Source: CAD feature listing. Evaluate the final solid. Frame: model axes, mm. Face numbers are marked on the shaded views. A direction names the side the tool comes from. Give positions to 0.01 mm unless a question says otherwise; leave off trailing zeros. Write each loop counter-clockwise with the first axis right and the second up, starting at its lowest first coordinate (ties: lowest second). Pieces come first, ordered by that corner, then holes. Notation, with made-up numbers: M 10,7 L 53,7 A12 cw 53,21 Z; hole C 58,-38 d4. An arc over 180 degrees is marked long. Answer as a JSON object with one key per item and string values. Group by question number.
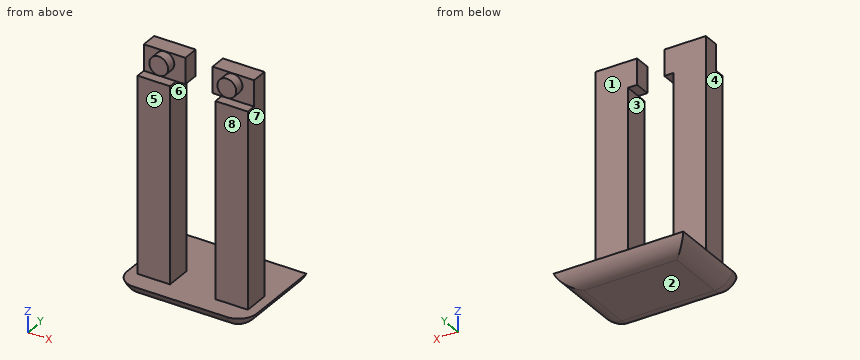
```python
from build123d import *

# Parameters (mm, degrees)
SKETCH1_W             = 50.8
SKETCH1_H             = 38.1
BOSS_EXTRUDE1_DEPTH   = 5.08
SKETCH2_W             = 16.51
SKETCH2_H             = 10.16
BOSS_EXTRUDE2_DEPTH   = 76.2
SKETCH3_W             = 3.81
SKETCH3_H             = 10.16
CUT_EXTRUDE1_DEPTH    = 76.2
SKETCH4_W             = 16.51
SKETCH4_H             = 10.16
BOSS_EXTRUDE3_DEPTH   = 12.7
SKETCH6_W             = 16.51
SKETCH6_H             = 12.7
CUT_EXTRUDE2_DEPTH    = 3.81
SKETCH5_R             = 3.683
BOSS_EXTRUDE4_DEPTH   = 3.81
FILLET1_R             = 7.62
FILLET4_R             = 7.62
FILLET7_R             = 7.62
SKETCH7_W             = 16.51
SKETCH7_H             = 6.35
LEDGE_REDUCTION_DEPTH = 2.54
SKETCH8_W             = 10.16
SKETCH8_H             = 6.35
CUT_EXTRUDE4_DEPTH    = 0.254
SKETCH9_W             = 10.16
SKETCH9_H             = 6.35
CUT_EXTRUDE5_DEPTH    = 0.254


with BuildPart() as part:
    # Sketch1 → Boss-Extrude1 (new body)
    with BuildSketch(Plane.XY):
        Rectangle(SKETCH1_W, SKETCH1_H)
    extrude(amount=BOSS_EXTRUDE1_DEPTH)

    # Sketch2 → Boss-Extrude2 (add)
    with BuildSketch(Plane.XY.offset(5.08)):
        with Locations((-13.335, -5.842)):
            Rectangle(SKETCH2_W, SKETCH2_H)
        with Locations((13.335, -5.842)):
            Rectangle(SKETCH2_W, SKETCH2_H)
    extrude(amount=BOSS_EXTRUDE2_DEPTH)

    # Sketch3 → Cut-Extrude1 (cut)
    with BuildSketch(Plane.XY.offset(81.28)):
        with Locations((-6.985, -5.842)):
            Rectangle(SKETCH3_W, SKETCH3_H)
        with Locations((6.985, -5.842)):
            Rectangle(SKETCH3_W, SKETCH3_H)
    extrude(amount=-CUT_EXTRUDE1_DEPTH, mode=Mode.SUBTRACT)

    # Sketch4 → Boss-Extrude3 (add)
    with BuildSketch(Plane.XY.offset(81.28)):
        with Locations((-13.335, -5.842)):
            Rectangle(SKETCH4_W, SKETCH4_H)
        with Locations((13.335, -5.842)):
            Rectangle(SKETCH4_W, SKETCH4_H)
    extrude(amount=BOSS_EXTRUDE3_DEPTH)

    # Sketch6 → Cut-Extrude2 (cut)
    with BuildSketch(Plane.XZ.offset(10.922)):
        with Locations((-13.335, 87.63)):
            Rectangle(SKETCH6_W, SKETCH6_H)
        with Locations((13.335, 87.63)):
            Rectangle(SKETCH6_W, SKETCH6_H)
    extrude(amount=-CUT_EXTRUDE2_DEPTH, mode=Mode.SUBTRACT)

    # Sketch5 → Boss-Extrude4 (add)
    with BuildSketch(Plane.XZ.offset(10.922)):
        with Locations(Location((-13.335, 87.63, 0), (0, 0, 270))):
            Circle(SKETCH5_R)
        with Locations(Location((13.335, 87.63, 0), (0, 0, 270))):
            Circle(SKETCH5_R)
    extrude(amount=-BOSS_EXTRUDE4_DEPTH)

    # Fillet1
    # the kernel refuses this fillet: 7.62 mm, written as the material it takes off along each edge
    with BuildSketch(Plane(origin=(-43.360512242, 19.05, 0), x_dir=(0, -1, 0), z_dir=(1, 0, 0))) as fillet1_piece_1:
        with BuildLine():
            CenterArc((7.184204897, -7.62), FILLET1_R, 90, 70.528779366)
            Line((0, -5.08), (-0.143684098, -5.0292))
            ThreePointArc((-0.143684098, -5.0292), (-0.1524, -2.54), (-0.1524, 0))
            Line((-0.1524, 0), (0, 0.1524))
            Line((0, 0.1524), (7.184204897, 0.1524))
            Line((7.184204897, 0.1524), (7.184204897, 0))
        make_face()
    extrude(amount=86.721024484, mode=Mode.SUBTRACT)

    # Fillet4
    # the kernel refuses this fillet: 7.62 mm, written as the material it takes off along each edge
    with BuildSketch(Plane(origin=(-25.4, -37.010512242, 0), x_dir=(0, 0, 1), z_dir=(0, 1, 0)), Plane(origin=(25.4, 29.826307345, 0), x_dir=(0, 0, 1), z_dir=(0, -1, 0))) as fillet4_piece_1:
        with BuildLine():
            CenterArc((7.62, 7.184204897), FILLET4_R, 180, 70.528779366)
            Line((0, 7.184204897), (-0.1524, 7.184204897))
            Line((-0.1524, 7.184204897), (-0.1524, 0))
            Line((-0.1524, 0), (0, -0.1524))
            ThreePointArc((0, -0.1524), (2.54, -0.1524), (5.0292, -0.143684098))
            Line((5.0292, -0.143684098), (5.08, 0))
        make_face()
    extrude(amount=66.836819587, mode=Mode.SUBTRACT)

    # Fillet7
    # the kernel refuses this fillet: 7.62 mm, written as the material it takes off along each edge
    with BuildSketch(Plane(origin=(-18.215795103, -19.05, 7.62), x_dir=(0.5563472554155052, 0, 0.8309498970405103), z_dir=(0.8309498970405103, 0, -0.5563472554155052))) as fillet7_piece_1:
        with BuildLine():
            CenterArc((7.62 - FILLET7_R, -FILLET7_R), FILLET7_R, 0, 90)
            Line((7.62, -FILLET7_R), (7.62, 0))
            Line((7.62, 0), (7.62 - FILLET7_R, 0))
        make_face()
    revolve(axis=Axis((-18.215795103, -19.05, 7.62), (0, -1, 0)), revolution_arc=213.803560609, mode=Mode.SUBTRACT)
    with BuildSketch(Plane(origin=(18.215795103, -19.05, 7.62), x_dir=(-0.5563472554155037, 0, 0.8309498970405114), z_dir=(-0.8309498970405114, 0, -0.5563472554155037))) as fillet7_piece_2:
        with BuildLine():
            CenterArc((7.62 - FILLET7_R, FILLET7_R), FILLET7_R, 270, 90)
            Line((7.62, FILLET7_R), (7.62, 0))
            Line((7.62, 0), (7.62 - FILLET7_R, 0))
        make_face()
    revolve(axis=Axis((18.215795103, -19.05, 7.62), (0, 1, 0)), revolution_arc=213.803560609, mode=Mode.SUBTRACT)
    with BuildSketch(Plane(origin=(18.215795103, -19.05, 0), x_dir=(0, 0, 1), z_dir=(-1, 0, 0))) as fillet7_piece_3:
        with BuildLine():
            CenterArc((FILLET7_R, FILLET7_R), FILLET7_R, 180, 90)
            Line((0, FILLET7_R), (0, 0))
            Line((0, 0), (FILLET7_R, 0))
        make_face()
    extrude(amount=36.431590206, mode=Mode.SUBTRACT)

    # Sketch7 → ledge-reduction (cut)
    with BuildSketch(Plane.XY.offset(93.98)):
        with Locations((-13.335, -3.937)):
            Rectangle(SKETCH7_W, SKETCH7_H)
        with Locations((13.335, -3.937)):
            Rectangle(SKETCH7_W, SKETCH7_H)
    extrude(amount=-LEDGE_REDUCTION_DEPTH, mode=Mode.SUBTRACT)

    # Sketch8 → Cut-Extrude4 (cut)
    with BuildSketch(Plane.ZY.offset(-5.08)):
        with Locations((86.36, -3.937)):
            Rectangle(SKETCH8_W, SKETCH8_H)
    extrude(amount=-CUT_EXTRUDE4_DEPTH, mode=Mode.SUBTRACT)

    # Sketch9 → Cut-Extrude5 (cut)
    with BuildSketch(Plane(origin=(-5.08, 0, 0), x_dir=(0, 0, -1), z_dir=(1, 0, 0))):
        with Locations((-86.36, -3.937)):
            Rectangle(SKETCH9_W, SKETCH9_H)
    extrude(amount=-CUT_EXTRUDE5_DEPTH, mode=Mode.SUBTRACT)


solid = part.part
```
(1) Section C-C, the plane y = -5. Return loops of the section in (x, z).
(2) Contact query for flat-ended pins moving along their axis: pin 1 Ø18 at (x, z) = (15.5, 53.5) entering from +Y; pin 2 Ø10 at (y, z) = (-12, 44) entering from +X; pin 3 Ø3 at (x, z) = (-11.5, 88.5) entering from -Y; pin 4 Ø8 at (x, z) = (3, 10) entering from -Y. Output: stop coordinate, or through.
(3) Section B-B, the plane z = 87.63. Return loops of the section in (x, y), plus the area to 3 significant figures.
(4) Section A-A, the plane x = 7.5. Return loops of the section in (y, z), plus the area to 3 significant figures.
(5) Ray query, L1, parallel to X at y = -7, z = 79; L2, parallel to Z at x = 1, y = -1.5; L3, parallel to Y at x = -20, z = 83.5. Return the intervals inside material, ascending. Write a range as [from, to].
(6) Access query for the marked faces 1, 2, 3, 4 and 5. Directions: +Z, -Z, +X, -X, +Y, -Y. A direction counts if a zero-diameter tool reaches every point of the face in a straight line with its end or side. Return the directions, or none.
(7) Section D-D, the plane z = 35.5. Return loops of the section in (x, y), plus the area to 3 significant figures.
(8) Pull-direction query (X, two-part tool) for the marked faces 6, 7 and 8; classes: pulls with the +X half, pulls with the -X half, needs draft (parallel to the pull), parting line crosses it, or undercut.
Reported:
{
 "1": {"outline": "M -25.4,5.08 A7.62 ccw -18.22,0 L 18.22,0 A7.62 ccw 25.4,5.08 L 21.59,5.08 L 21.59,91.44 L 5.33,91.44 L 5.33,81.28 L 8.89,81.28 L 8.89,5.08 L -8.89,5.08 L -8.89,81.28 L -5.33,81.28 L -5.33,91.44 L -21.59,91.44 L -21.59,5.08 Z"},
 "2": {"pin 1": "stops at y = -0.76", "pin 2": "stops at x = 21.59", "pin 3": "stops at y = -10.92", "pin 4": "passes through"},
 "3": {"outline": "M -21.59,-7.11 L -17.02,-7.11 L -17.02,-10.92 L -9.65,-10.92 L -9.65,-7.11 L -5.33,-7.11 L -5.33,-0.76 L -21.59,-0.76 Z; M 5.33,-7.11 L 9.65,-7.11 L 9.65,-10.92 L 17.02,-10.92 L 17.02,-7.11 L 21.59,-7.11 L 21.59,-0.76 L 5.33,-0.76 Z", "area": "263 mm2"},
 "4": {"outline": "M -18.61,5.08 A7.62 ccw -11.43,0 L 11.87,0 A7.62 ccw 19.05,5.08 Z; M -7.11,81.28 L -0.76,81.28 L -0.76,91.44 L -7.11,91.44 Z", "area": "236 mm2"},
 "5": {"L1": "x = [-21.59, -8.89], [8.89, 21.59]", "L2": "z = [0, 5.08]", "L3": "y = [-7.11, -0.76]"},
 "6": {"face 1": "+Z, +X, -X, +Y", "face 2": "-Z, +X, -X, +Y, -Y", "face 3": "+Y, -Y", "face 4": "+Z, -X, +Y, -Y", "face 5": "+Z, +X, -X, -Y"},
 "7": {"outline": "M -21.59,-10.92 L -8.89,-10.92 L -8.89,-0.76 L -21.59,-0.76 Z; M 8.89,-10.92 L 21.59,-10.92 L 21.59,-0.76 L 8.89,-0.76 Z", "area": "258 mm2"},
 "8": {"face 6": "undercut", "face 7": "pulls with the +X half", "face 8": "needs draft"}
}
